Print and shaded views of the part. All mm, measured from the part's lowest x, y and z. Round coordinates to 2 decimals unless told otherwise and drop trailing zeros. Order: outer loops, then holes, each group sorted by start corner. A loop starts at its lowest first (then second) coordinate and runs counter-clockwise, first axis right, second up. Notation, with made-up numbers: (31.25, 68) -> (69.25, 68) arc R21 cw to (69.25, 95) -> close; hole circle Ø10 at (25.5, 27). An arc over 180 degrees is marked (long way). Answer as CSV lines item,"result".
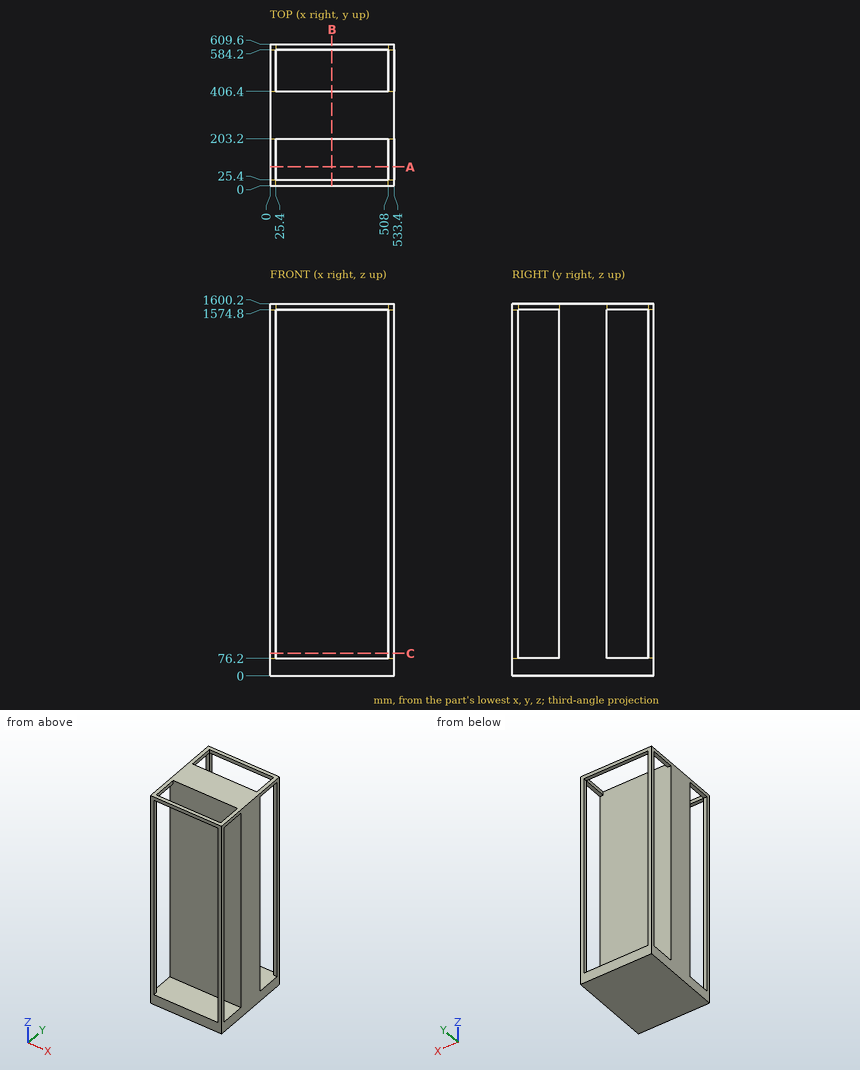
Q1. Saw through at B-B (x = 265.5). Write the cut outline in (y, z), plus the area to 3 significant figures.
Checks:
outline,"(0, 0) -> (609.6, 0) -> (609.6, 76.2) -> (406.4, 76.2) -> (406.4, 1600.2) -> (203.2, 1600.2) -> (203.2, 76.2) -> (0, 76.2) -> close; (0, 1574.8) -> (25.4, 1574.8) -> (25.4, 1600.2) -> (0, 1600.2) -> close; (584.2, 1574.8) -> (609.6, 1574.8) -> (609.6, 1600.2) -> (584.2, 1600.2) -> close"
area,"357,000 mm²"
Q2. Flat gauge pin, fed straight in: pin 1 (8 mm diameter, centred on x = 138.5, z = 432, fed in from -Y). Where does the tip first touch, or does it go through?
Checks:
pin 1,"y = 203.2"
Q3. Saw through at A-A (y = 81.5). Write the cut outline in (x, z), plus the area to 3 significant figures.
Checks:
outline,"(0, 0) -> (533.4, 0) -> (533.4, 76.2) -> (0, 76.2) -> close; (0, 1574.8) -> (25.4, 1574.8) -> (25.4, 1600.2) -> (0, 1600.2) -> close; (508, 1574.8) -> (533.4, 1574.8) -> (533.4, 1600.2) -> (508, 1600.2) -> close"
area,"41,900 mm²"
Q4. Wall check: L1, parallel to Y at x = 509, z = 975; L2, parallel to Y at x = 268.5, z = 689; L3, parallel to Z at x = 176, y = 112. Give the ranges that are in metal, low to high. Write a range as [from, to].
Checks:
L1,"[0, 25.4], [203.2, 406.4], [584.2, 609.6]"
L2,"[203.2, 406.4]"
L3,"[0, 76.2]"
Q5. Saw through at C-C (z = 97.5). Write the cut outline in (x, y).
Checks:
outline,"(0, 0) -> (25.4, 0) -> (25.4, 25.4) -> (0, 25.4) -> close; (0, 203.2) -> (533.4, 203.2) -> (533.4, 406.4) -> (0, 406.4) -> close; (0, 584.2) -> (25.4, 584.2) -> (25.4, 609.6) -> (0, 609.6) -> close; (508, 0) -> (533.4, 0) -> (533.4, 25.4) -> (508, 25.4) -> close; (508, 584.2) -> (533.4, 584.2) -> (533.4, 609.6) -> (508, 609.6) -> close"
